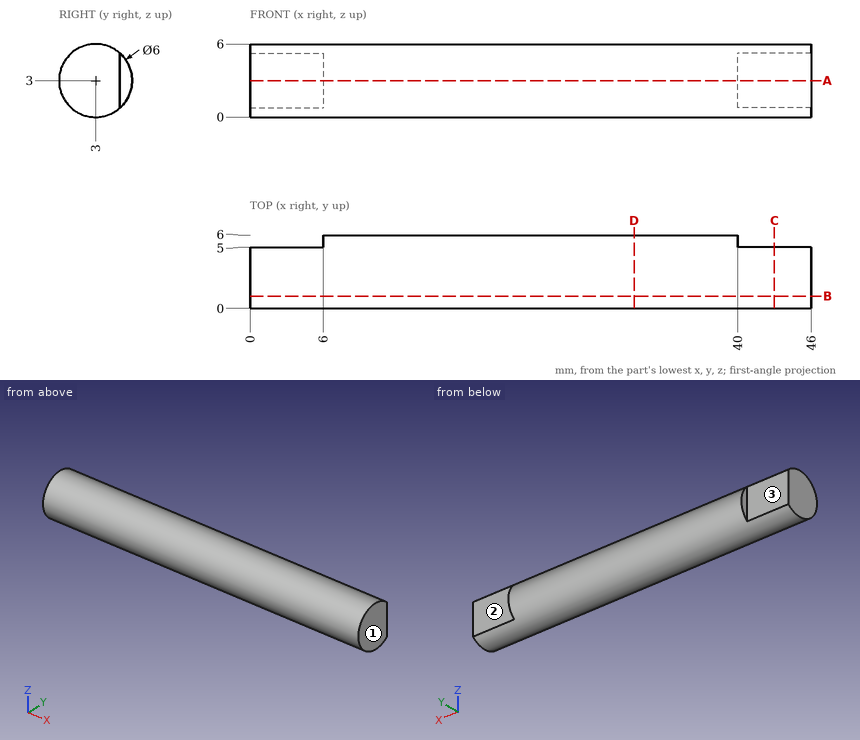
Answer from the drawing. Dimensions are ordinates in mm from the lowest x, y and z of the part. A direction names the side the tool comes from. Coordinates: 2 decimals unless noted, no trailing zeros. Order: outer loops, then holes, each group sorted by start corner. A loop starts at its lowest first (then second) coordinate and runs counter-clockwise, first axis right, second up. Notation, with made-up numbers: (77.5, -16.5) - (87.5, -16.5) arc R21 ccw to (87.5, -1.5) - close; hole circle Ø5 at (-38, 29.25). An arc over 180 degrees is marked (long way). Answer as a JSON object with one key per item and string values. Group by question number.
Item 1: Section A-A (z = 3) is taken. Give the vertices of the cut face in (x, y), plus the area to 3 significant figures.
Item 2: Consider probe 1 along X at (y, z) = (5.25, 3.7); probe 2 along Z at (x, y) = (11, 5); probe 3 along Z at (x, y) = (16, 3.25). Determine where each line is inside the solid, lowest interval first. Write a range as from..to.
Item 3: A tool of negligible diameter and unlimited length cuts with its end or side. For the marked faces 1, 2 and 3, from which of +Z, -Z, +X, -X, +Y, -Y can it reach the whole face along a straight path? Write none if from no direction.
Item 4: Flat-ended cylindrical pins translate along their axes: P1, Ø0.5, axis at y = 5.5, z = 3, coming from the -X side; P2, Ø1.3, axis at x = 2.5, z = 3, coming from the +Y side; P3, Ø1.5, axis at x = 20, z = 4.5, coming from the +Y side. Find the tip coordinate at first contact, or state that the pin passes through.
Item 5: Section B-B (y = 1) is taken. Give the vertices of the cut face in (x, z).
Item 6: Section D-D (x = 31.5) is taken. Give the vertices of the cut face in (y, z).
Item 7: Section C-C (x = 43) is taken. Give the vertices of the cut face in (y, z), plus the area to 3 significant figures.
Results are:
{
 "1": {"outline": "(0, 0) - (46, 0) - (46, 5) - (40, 5) - (40, 6) - (6, 6) - (6, 5) - (0, 5) - close", "area": "264 mm^2"},
 "2": {"probe 1": "x = 6..40", "probe 2": "z = 0.76..5.24", "probe 3": "z = 0.01..5.99"},
 "3": {"face 1": "+Z, -Z, +X, +Y, -Y", "face 2": "+Z, -Z, +X, +Y", "face 3": "+Z, -Z, -X, +Y"},
 "4": {"P1": "stops at x = 6", "P2": "stops at y = 5", "P3": "stops at y = 5.9"},
 "5": {"outline": "(0, 0.76) - (46, 0.76) - (46, 5.24) - (0, 5.24) - close"},
 "6": {"outline": "circle Ø6 at (3, 3)"},
 "7": {"outline": "(5, 0.76) - (5, 5.24) arc R3 ccw (long way) to start", "area": "25.2 mm^2"}
}
